Read the model definition and answer for the solid it produces. Units are mm, in the model's axes. A direction names the side the tool comes from. Coordinates: 2 decimals unless noted, no trailing zeros. Write each loop counter-clockwise with the first axis right and the second up, starting at its lowest first coordinate (ties: lowest second). Pieces come first, ordered by that corner, then holes.
(1) Find the intervals of material crossed by probe 1 along Y at (x, z) = (-1.65, -3); probe 2 along Y at (x, z) = (-0.4, -46); probe 3 along Z at (x, y) = (-2.2, -0.5), in increasing order.
(2) Section C-C on x = -0.6 is taken. Write down the section's boundary in (y, z), then the cut area to 3 significant figures.
(3) The mould has two halves that part along Z. Classify faces 1 (the flat face through (-4, 27, -29)), 2 (the flat face through (-2, 30, -58)), 3 (the cylindrical face through (-2, 3, -54)), 4 (the flat face through (-2, -2, -26.5)): +Z half, -Z half, draft (parallel to the pull), parting line (faces both ways), or undercut.
(4) Section B-B on y = 3 is taken. Write down the section's boundary in (x, z), then the cut area to 3 significant figures.
(5) Which of the six approach directions +Z, -Z, +X, -X, +Y, -Y give full straight-line access (tool end or side, diameter ignored) to faces 5 (the flat face through (-2, -2, -31.5)), 6 (the flat face through (0, 27, -29)), 7 (the flat face through (-2, 0, -13))?
(6) Section A-A on z = -3 is taken. Write down the section's boundary in (x, y), then the cut area to 3 significant figures.
Autodesk Inventor part; units mm, degrees
ref_plane "YZ Plane" through (0, 0, 0) normal (1, 0, 0) x (0, 1, 0)
ref_plane "XZ Plane" through (0, 0, 0) normal (0, 1, 0) x (-1, 0, 0)
ref_plane "XY Plane" through (0, 0, 0) normal (0, 0, 1) x (1, 0, 0)
sketch "Sketch1" plane through (0, 0, 0) normal (0, 1, 0) x (-1, 0, 0)
  line L0 (0, 0) -> (4, 0)
  line L1 (4, 0) -> (4, -58)
  line L2 (4, -58) -> (0, -58)
  line L3 (0, -58) -> (0, 0)
  dimension "d0" = 58
  dimension "d1" = 4
extrude "Extrusion1" add sketch "Sketch1" along normal blind 60
sketch "Sketch2" plane through (-4, 0, 0) normal (0, 0, 1) x (1, 0, 0)
  circle A0 centre (2, 2) radius 1
  line L0 (4, 0) -> (0, 0)
  line L1 (4, 0) -> (4, 60)
  dimension "d4" = 2
  dimension "d5" = 2
  dimension "d6" = 2
extrude "Extrusion2" [suppressed]
fillet "Fillet1" [suppressed]
sketch "Sketch3" plane through (0, 2, 0) normal (1, 0, 0) x (0, 0, -1)
  line L0 (19, 20.5) -> (24, 20.5)
  line L1 (24, 20.5) -> (24, 35.5)
  line L2 (24, 35.5) -> (19, 35.5)
  line L3 (19, 35.5) -> (19, 20.5)
  line L4 (34, 20.5) -> (39, 20.5)
  line L5 (39, 20.5) -> (39, 35.5)
  line L6 (39, 35.5) -> (34, 35.5)
  line L7 (34, 35.5) -> (34, 20.5)
  line L8 (0, -2) -> (0, 58)
  line L9 (58, -2) -> (58, 58)
  line L10 (0, -2) -> (58, -2)
  line L11 (0, 58) -> (58, 58)
  point P0 (0, 0)
  point P1 (0, 56)
  point P2 (58, 0)
  point P3 (58, 56)
  dimension "d10" = 15
  dimension "d11" = 15
  dimension "d12" = 5
  dimension "d13" = 5
  dimension "d14" = 10
  dimension "d15" = 19
  dimension "d16" = 58
  dimension "d17" = 60
  dimension "d18" = 22.5
extrude "Extrusion3" [suppressed]
sketch "Sketch4" plane through (0, 22.5, -19) normal (0, 0, 1) x (1, 0, 0)
  circle A0 centre (5, 7.5) radius 1.5
  line L0 (0, 0) -> (10, 0)
  line L1 (10, 0) -> (10, 15)
  point P0 (0, -22.5)
  dimension "d21" = 3
  dimension "d22" = 7.5
  dimension "d23" = 5
  dimension "d24" = 15
  dimension "d25" = 10
extrude "Extrusion4" [suppressed]
fillet "Fillet2" [suppressed]
sketch "Esquisse5" plane through (0, 0, 0) normal (1, 0, 0) x (0, 0, -1)
  circle A0 centre (55, 3) radius 1
  circle A1 centre (3, 3) radius 1
  line L0 (0, 0) -> (0, 60)
  line L1 (58, 0) -> (0, 0)
  line L2 (58, 0) -> (58, 60)
  dimension "d29" = 2
  dimension "d30" = 2
  dimension "d31" = 3
  dimension "d32" = 3
  dimension "d33" = 3
  dimension "d34" = 3
extrude "Extrusion5" cut sketch "Esquisse5" against normal blind 10
sketch "Esquisse6" plane through (0, 0, 0) normal (0, -1, 0) x (1, 0, 0)
  line L0 (-4, -58) -> (-4, 0)
  line L1 (0, 0) -> (0, -58)
  line L2 (-4, -26.5) -> (0, -26.5)
  line L3 (0, -26.5) -> (0, -31.5)
  line L4 (0, -31.5) -> (-4, -31.5)
  line L5 (-4, -31.5) -> (-4, -26.5)
  line L6 (0, 0) -> (-4, 0)
  dimension "d37" = 5
  dimension "d38" = 26.5
  dimension "d39" = 58
extrude "Extrusion6" add sketch "Esquisse6" along normal blind 5 contours L0 L2 L1 L4
equation "\"d6\" = d5"
equation "\"d11\" = d10"
equation "\"d13\" = d12"
equation "\"d15\" = 0.5 * d16 - 0.5 * d14 - 0.5 * d12 - 0.5 * d13"
equation "\"d18\" = 0.5 * d17 - 0.5 * d10"
equation "\"d22\" = 0.5 * d24"
equation "\"d23\" = 0.5 * d25"
equation "\"d32\" = d31"
equation "\"d33\" = d32"
equation "\"d34\" = d33"
equation "\"d38\" = 0.5 * d39 - 0.5 * d37"
properties part number "extremite_pince" material "PC/ABS Plastic"
Response:
1. probe 1: y = 0 to 2, 4 to 60
1. probe 2: y = 0 to 60
1. probe 3: z = -31.5 to -26.5
2. outline: (-5, -31.5) - (0, -31.5) - (0, -58) - (60, -58) - (60, 0) - (0, 0) - (0, -26.5) - (-5, -26.5) - close; hole circle Ø2 at (3, -55); hole circle Ø2 at (3, -3)
2. area: 3,500 mm2
3. face 1: draft
3. face 2: -Z half
3. face 3: undercut
3. face 4: +Z half
4. outline: (-4, -58) - (0, -58) - (0, -56) - (-4, -56) - close; (-4, -54) - (0, -54) - (0, -4) - (-4, -4) - close; (-4, -2) - (0, -2) - (0, 0) - (-4, 0) - close
4. area: 216 mm2
5. face 5: -Z, +X, -X, -Y
5. face 6: +Z, -Z, +X, +Y, -Y
5. face 7: +Z, +X, -X, -Y
6. outline: (-4, 0) - (0, 0) - (0, 2) - (-4, 2) - close; (-4, 4) - (0, 4) - (0, 60) - (-4, 60) - close
6. area: 232 mm2
